Source: CAD feature listing. Evaluate the final solid. Frame: model axes, mm. A direction names the side the tool comes from. Round coordinates to 2 decimals unless told otherwise and drop trailing zeros. Loops run counter-clockwise (first coordinate to the right, second up) from the corner with the lowest first, then second, coordinate; pieces in that order, holes last. Notation, with made-up numbers: M 26.5,71 L 39.5,71 A22 cw 39.5,81 Z; hole C 19,10.5 d8. An arc over 180 degrees is marked long. Answer as a JSON object with one key per item and string values.
from build123d import *

# Parameters (mm, degrees)
BOX001_W            = 126
BOX001_H            = 23
BOX001_DEPTH        = 3
HOLE003_D           = 3.4
HOLE003_DEPTH       = 24
HOLE003_CBORE_D     = 6
HOLE003_CBORE_DEPTH = 2.1
POCKET_DEPTH        = 1
POCKET001_DEPTH     = 5
CHAMFER_SIZE2       = 2.09
CHAMFER_SIZE        = 1
FILLET001_R         = 5
CHAMFER001_SIZE2    = 14
CHAMFER001_SIZE     = 28
CHAMFER002_SIZE2    = 14
CHAMFER002_SIZE     = 28
FILLET002_R         = 5
FILLET003_R         = 30


with BuildPart() as part:
    # Box001 → Box001 (join)
    with BuildSketch(Plane.XY):
        with Locations((63, 11.5)):
            Rectangle(BOX001_W, BOX001_H)
    extrude(amount=BOX001_DEPTH)

    # Hole003
    with Locations(Plane.XY.offset(3)):
        with Locations((5, 5), (58, 5), (68, 5), (121, 5)):
            CounterBoreHole(HOLE003_D / 2, HOLE003_CBORE_D / 2, HOLE003_CBORE_DEPTH, depth=HOLE003_DEPTH)

    # Sketch006 (on Face5 of Hole003) → Pocket (cut)
    with BuildSketch(Plane(origin=(0, 0, 0), x_dir=(1, 0, 0), z_dir=(0, 0, -1))):
        with BuildLine():
            ThreePointArc((34.5, -12.5), (31, -16), (34.5, -19.5))
            Line((34.5, -19.5), (91.5, -19.5))
            ThreePointArc((91.5, -19.5), (95, -16), (91.5, -12.5))
            Line((34.5, -12.5), (91.5, -12.5))
        make_face()
    extrude(amount=-POCKET_DEPTH, mode=Mode.SUBTRACT)

    # Sketch007 (on Face23 of Pocket) → Pocket001 (cut)
    with BuildSketch(Plane(origin=(0, 0, 1), x_dir=(1, 0, 0), z_dir=(0, 0, -1))):
        with BuildLine():
            ThreePointArc((34.5, -14.25), (32.75, -16), (34.5, -17.75))
            Line((34.5, -17.75), (91.5, -17.75))
            ThreePointArc((91.5, -17.75), (93.25, -16), (91.5, -14.25))
            Line((34.5, -14.25), (91.5, -14.25))
        make_face()
    extrude(amount=-POCKET001_DEPTH, mode=Mode.SUBTRACT)

    # Chamfer
    chamfer_edges = [part.edges().sort_by_distance(p)[0] for p in [
        (2, 5, 3),
        (55, 5, 3),
        (65, 5, 3),
        (118, 5, 3),
    ]]
    chamfer_side = part.faces().sort_by_distance((63, 11.420058, 3))[0]
    chamfer(chamfer_edges, length=CHAMFER_SIZE, length2=CHAMFER_SIZE2, reference=chamfer_side)

    # Fillet001
    fillet001_edges = [part.edges().sort_by_distance(p)[0] for p in [
        (0, 0, 1.5),
        (126, 0, 1.5),
    ]]
    fillet(fillet001_edges, radius=FILLET001_R)

    # Chamfer001
    chamfer001_edges = [part.edges().sort_by_distance(p)[0] for p in [
        (126, 23, 1.5),
    ]]
    chamfer001_side = part.faces().sort_by_distance((63, 23, 1.5))[0]
    chamfer(chamfer001_edges, length=CHAMFER001_SIZE, length2=CHAMFER001_SIZE2, reference=chamfer001_side)

    # Chamfer002
    chamfer002_edges = [part.edges().sort_by_distance(p)[0] for p in [
        (0, 23, 1.5),
    ]]
    chamfer002_side = part.faces().sort_by_distance((49, 23, 1.5))[0]
    chamfer(chamfer002_edges, length=CHAMFER002_SIZE, length2=CHAMFER002_SIZE2, reference=chamfer002_side)

    # Fillet002
    fillet002_edges = [part.edges().sort_by_distance(p)[0] for p in [
        (0, 9, 1.5),
        (126, 9, 1.5),
    ]]
    fillet(fillet002_edges, radius=FILLET002_R)

    # Fillet003
    fillet003_edges = [part.edges().sort_by_distance(p)[0] for p in [
        (28, 23, 1.5),
        (98, 23, 1.5),
    ]]
    fillet(fillet003_edges, radius=FILLET003_R)


solid = part.part
Item 1: Section D-D on x = 17.5. Return the cut outline in (y, z).
Answer sheet:
{"outline": "M 0,0 L 17.75,0 L 17.75,3 L 0,3 Z"}
Item 2: Section C-C on z = 2.15. Return the cut outline in (x, y).
Answer sheet:
{"outline": "M 0,5 A5 ccw 5,0 L 121,0 A5 ccw 126,5 L 126,5.91 A5 ccw 123.24,10.38 L 104.33,19.83 A30 ccw 90.92,23 L 35.08,23 A30 ccw 21.67,19.83 L 2.76,10.38 A5 ccw 0,5.91 Z; hole C 5,5 d7.19; hole M 34.5,14.25 L 91.5,14.25 A1.75 ccw 91.5,17.75 L 34.5,17.75 A1.75 ccw Z; hole C 58,5 d7.19; hole C 68,5 d7.19; hole C 121,5 d7.19"}
Item 3: Pull-direction query (Y, two-part tool) for faces 4 (the flat face through (62, 0, 1)), 5 (the flat face through (63, 14.25, 2)), 6 (the flat face through (63, 14, 1)), 7 (the cylindrical face through (0.767, 8.571, 1.521)); classes: pulls with the +Y half, pulls with the -Y half, needs draft (parallel to the pull), parting line crosses it, or undercut.
Answer sheet:
{"face 4": "pulls with the -Y half", "face 5": "undercut", "face 6": "undercut", "face 7": "pulls with the +Y half"}
Item 4: Section A-A on y = 16. Return the cut outline in (x, z).
Answer sheet:
{"outline": "M 14,0 L 31,0 L 31,1 L 32.75,1 L 32.75,3 L 14,3 Z; M 93.25,1 L 95,1 L 95,0 L 112,0 L 112,3 L 93.25,3 Z"}
Item 5: Access query for faces 1 (the flat face through (5, 3, 0.9)), 2 (the flat face through (114, 15, 1)), 3 (the flat face through (63, 17.75, 2)). Directions: +Z, -Z, +X, -X, +Y, -Y. A direction counts if a zero-diameter tool reaches every point of the face in a straight line with its end or side. Return the directions, or none.
Answer sheet:
{"face 1": "+Z", "face 2": "+Z, -Z, +X, +Y", "face 3": "+Z, -Z"}
Item 6: Line query: probe 1 along Y at (x, z) = (68, 0.4); probe 2 along Y at (x, z) = (58, 0.95); probe 3 along X at (y, z) = (5, 0.95). Output: solid intervals per line, ascending. Write a range as from..to.
Answer sheet:
{"probe 1": "y = 0..3.3, 6.7..12.5, 19.5..23", "probe 2": "y = 0..1.98, 8.02..12.5, 19.5..23", "probe 3": "x = 0..1.98, 8.02..54.98, 61.02..64.98, 71.02..117.98, 124.02..126"}
Item 7: Contact query for flat-ended pins moving along their axis: pin 1 Ø2 at (x, y) = (68, 5) entering from -Z; pin 2 Ø3.5 at (x, y) = (58, 5) entering from +Z; pin 3 Ø3.5 at (x, y) = (76, 16.5) entering from -Z; pin 4 Ø7 at (x, y) = (121, 5) entering from +Z (3 decimals). Output: stop coordinate, or through.
Answer sheet:
{"pin 1": "passes through", "pin 2": "stops at z = 0.9", "pin 3": "stops at z = 1", "pin 4": "stops at z = 1.955"}
Item 8: Section B-B on x = 58. Give the number of separate pieces and of enclosed holes in the cut face, then the cut area to 4 significant figures.
Answer sheet:
{"separate pieces": "3", "enclosed holes": "0", "area": "37.25 mm²"}
